Could you check a few things on this model? Use its own coordinates, in mm. Face numbers are marked on the shaded views. A direction names the side the tool comes from. Coordinates: 2 decimals unless noted, no trailing zeros. Loops run counter-clockwise (first coordinate to the right, second up) from the corner with the lowest first, then second, coordinate; pieces in that order, holes last. Notation, with made-up numbers: (16.5, 88.25) -> (40.5, 88.25) arc R15 ccw to (40.5, 98.25) -> close; hole circle Ø4 at (26, 0.5). An arc over 180 degrees is marked (long way). One line per question, with ' | ' between items. Start each with the question number.
(1) If we mould it in two halves opening along Z, with no side actions, what happens to the marked faces 1, 2 and 3? For each: pulls with the +Z half, pulls with the -Z half, needs draft (parallel to the pull), parting line crosses it, or undercut.
(2) Which directions (+Z, -Z, +X, -X, +Y, -Y) give clear straight access to the entire face, cutting with the end or side of a thin tool? Please do the marked faces 4 and 5.
(3) Suppose I cut it at B-B (y = 0). Please give me the cut outline in (x, z), plus the area to 3 significant figures.
(4) If I drill on line 1 along Z through (x, y) = (35.5, -33); line 2 along Z through (x, y) = (24.5, 41.5); line 3 along Y through (x, z) = (26.5, -79), over which ranges is the centre line in solid material (lowest first)?
(5) Suppose I cut it at A-A (x = 30). Give the number of separate pieces and of enclosed holes in the cut face, plus the area to 3 significant figures.
(6) I'm going to push flat-ended pins straight in: pin 1 Ø4 at (x, z) = (39.5, 85) entering from +Y; pin 2 Ø3 at (y, z) = (-20, 96) entering from -X; pin 3 Ø6 at (x, y) = (30.5, 65.5) entering from +Z; pin 4 Ø11 at (x, z) = (6.5, 47.5) entering from +Y. Where does each tip first touch, or does it pass through?
```python
from build123d import *

# Parameters (mm, degrees)
CUT_EXTRUDE1_START = -10
CUT_EXTRUDE1_DEPTH = 214.774440026
CUT_EXTRUDE2_DEPTH = 224.774440026


with BuildPart() as part:
    # Çizim1 → Döndür1 (revolve)
    with BuildSketch(Plane.XY, mode=Mode.PRIVATE) as d_nd_r1_sk:
        with BuildLine():
            Line((0, 31), (5, 31))
            Line((5, 31), (5, 32.75))
            Line((5, 32.75), (7.3, 32.75))
            Line((7.3, 32.75), (7.3, 31))
            Line((7.3, 31), (25, 31))
            Line((25, 31), (25, 16))
            Line((25, 16), (35, 16))
            Line((35, 16), (35, 0))
            Line((35, 0), (45, 0))
            Line((45, 0), (45, 148.5))
            Line((45, 148.5), (45, 150))
            ThreePointArc((45, 150), (43.535533906, 153.535533906), (40, 155))
            Line((40, 155), (25, 155))
            Line((25, 155), (25, 135))
            Line((25, 135), (5, 135))
            Line((5, 135), (0, 133))
            Line((0, 133), (0, 31))
        make_face()
    revolve(d_nd_r1_sk.sketch.rotate(Axis((0, 0, 0), (1, 0, 0)), 90), axis=Axis((0, 0, 0), (1, 0, 0)))

    # Sketch2 → Cut-Extrude1 (cut, through all)
    with BuildSketch(Plane.ZY.offset(CUT_EXTRUDE1_START)):
        with BuildLine():
            Line((82.068542495, 87.068542495), (31.068542495, 87.068542495))
            ThreePointArc((31.068542495, 87.068542495), (27.533008589, 85.604076401), (26.068542495, 82.068542495))
            Line((26.068542495, 82.068542495), (26.068542495, 31.068542495))
            ThreePointArc((26.068542495, 31.068542495), (27.533008589, 27.533008589), (31.068542495, 26.068542495))
            Line((31.068542495, 26.068542495), (82.068542495, 26.068542495))
            ThreePointArc((82.068542495, 26.068542495), (85.604076401, 27.533008589), (87.068542495, 31.068542495))
            Line((87.068542495, 31.068542495), (87.068542495, 82.068542495))
            ThreePointArc((87.068542495, 82.068542495), (85.604076401, 85.604076401), (82.068542495, 87.068542495))
        make_face()
        with BuildLine():
            Line((-82.068542495, 87.068542495), (-31.068542495, 87.068542495))
            ThreePointArc((-31.068542495, 87.068542495), (-27.533008589, 85.604076401), (-26.068542495, 82.068542495))
            Line((-26.068542495, 82.068542495), (-26.068542495, 31.068542495))
            ThreePointArc((-26.068542495, 31.068542495), (-27.533008589, 27.533008589), (-31.068542495, 26.068542495))
            Line((-31.068542495, 26.068542495), (-82.068542495, 26.068542495))
            ThreePointArc((-82.068542495, 26.068542495), (-85.604076401, 27.533008589), (-87.068542495, 31.068542495))
            Line((-87.068542495, 31.068542495), (-87.068542495, 82.068542495))
            ThreePointArc((-87.068542495, 82.068542495), (-85.604076401, 85.604076401), (-82.068542495, 87.068542495))
        make_face()
        with BuildLine():
            Line((87.068542495, -82.068542495), (87.068542495, -31.068542495))
            ThreePointArc((87.068542495, -31.068542495), (85.604076401, -27.533008589), (82.068542495, -26.068542495))
            Line((82.068542495, -26.068542495), (31.068542495, -26.068542495))
            ThreePointArc((31.068542495, -26.068542495), (27.533008589, -27.533008589), (26.068542495, -31.068542495))
            Line((26.068542495, -31.068542495), (26.068542495, -82.068542495))
            ThreePointArc((26.068542495, -82.068542495), (27.533008589, -85.604076401), (31.068542495, -87.068542495))
            Line((31.068542495, -87.068542495), (82.068542495, -87.068542495))
            ThreePointArc((82.068542495, -87.068542495), (85.604076401, -85.604076401), (87.068542495, -82.068542495))
        make_face()
        with BuildLine():
            Line((-82.068542495, -87.068542495), (-31.068542495, -87.068542495))
            ThreePointArc((-31.068542495, -87.068542495), (-27.533008589, -85.604076401), (-26.068542495, -82.068542495))
            Line((-26.068542495, -82.068542495), (-26.068542495, -31.068542495))
            ThreePointArc((-26.068542495, -31.068542495), (-27.533008589, -27.533008589), (-31.068542495, -26.068542495))
            Line((-31.068542495, -26.068542495), (-82.068542495, -26.068542495))
            ThreePointArc((-82.068542495, -26.068542495), (-85.604076401, -27.533008589), (-87.068542495, -31.068542495))
            Line((-87.068542495, -31.068542495), (-87.068542495, -82.068542495))
            ThreePointArc((-87.068542495, -82.068542495), (-85.604076401, -85.604076401), (-82.068542495, -87.068542495))
        make_face()
    extrude(amount=-CUT_EXTRUDE1_DEPTH, mode=Mode.SUBTRACT)

    # Sketch4 → Cut-Extrude2 (cut, through all)
    with BuildSketch(Plane.ZY):
        with BuildLine():
            Line((36.068542495, -31.068542495), (77.068542495, -31.068542495))
            ThreePointArc((77.068542495, -31.068542495), (80.604076401, -32.533008589), (82.068542495, -36.068542495))
            Line((82.068542495, -36.068542495), (82.068542495, -77.068542495))
            ThreePointArc((82.068542495, -77.068542495), (80.604076401, -80.604076401), (77.068542495, -82.068542495))
            Line((77.068542495, -82.068542495), (36.068542495, -82.068542495))
            ThreePointArc((36.068542495, -82.068542495), (32.533008589, -80.604076401), (31.068542495, -77.068542495))
            Line((31.068542495, -77.068542495), (31.068542495, -36.068542495))
            ThreePointArc((31.068542495, -36.068542495), (32.533008589, -32.533008589), (36.068542495, -31.068542495))
        make_face()
        with BuildLine():
            Line((-36.068542495, -31.068542495), (-77.068542495, -31.068542495))
            ThreePointArc((-77.068542495, -31.068542495), (-80.604076401, -32.533008589), (-82.068542495, -36.068542495))
            Line((-82.068542495, -36.068542495), (-82.068542495, -77.068542495))
            ThreePointArc((-82.068542495, -77.068542495), (-80.604076401, -80.604076401), (-77.068542495, -82.068542495))
            Line((-77.068542495, -82.068542495), (-36.068542495, -82.068542495))
            ThreePointArc((-36.068542495, -82.068542495), (-32.533008589, -80.604076401), (-31.068542495, -77.068542495))
            Line((-31.068542495, -77.068542495), (-31.068542495, -36.068542495))
            ThreePointArc((-31.068542495, -36.068542495), (-32.533008589, -32.533008589), (-36.068542495, -31.068542495))
        make_face()
        with BuildLine():
            Line((-31.068542495, 36.068542495), (-31.068542495, 77.068542495))
            ThreePointArc((-31.068542495, 77.068542495), (-32.533008589, 80.604076401), (-36.068542495, 82.068542495))
            Line((-36.068542495, 82.068542495), (-77.068542495, 82.068542495))
            ThreePointArc((-77.068542495, 82.068542495), (-80.604076401, 80.604076401), (-82.068542495, 77.068542495))
            Line((-82.068542495, 77.068542495), (-82.068542495, 36.068542495))
            ThreePointArc((-82.068542495, 36.068542495), (-80.604076401, 32.533008589), (-77.068542495, 31.068542495))
            Line((-77.068542495, 31.068542495), (-36.068542495, 31.068542495))
            ThreePointArc((-36.068542495, 31.068542495), (-32.533008589, 32.533008589), (-31.068542495, 36.068542495))
        make_face()
        with BuildLine():
            Line((36.068542495, 31.068542495), (77.068542495, 31.068542495))
            ThreePointArc((77.068542495, 31.068542495), (80.604076401, 32.533008589), (82.068542495, 36.068542495))
            Line((82.068542495, 36.068542495), (82.068542495, 77.068542495))
            ThreePointArc((82.068542495, 77.068542495), (80.604076401, 80.604076401), (77.068542495, 82.068542495))
            Line((77.068542495, 82.068542495), (36.068542495, 82.068542495))
            ThreePointArc((36.068542495, 82.068542495), (32.533008589, 80.604076401), (31.068542495, 77.068542495))
            Line((31.068542495, 77.068542495), (31.068542495, 36.068542495))
            ThreePointArc((31.068542495, 36.068542495), (32.533008589, 32.533008589), (36.068542495, 31.068542495))
        make_face()
    extrude(amount=-CUT_EXTRUDE2_DEPTH, mode=Mode.SUBTRACT)


solid = part.part
```
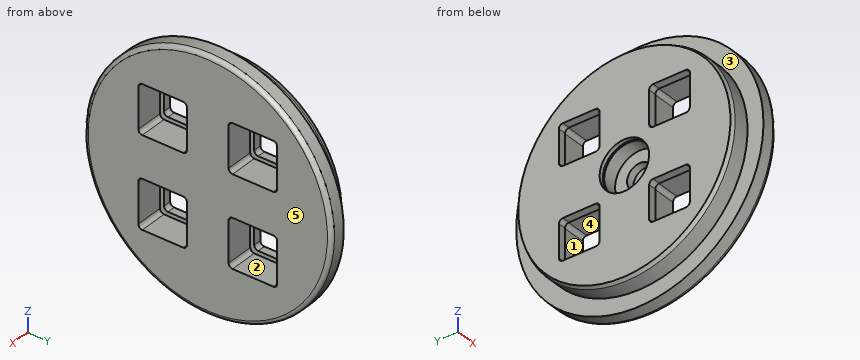
Checks:
1) face 1: undercut | face 2: undercut | face 3: needs draft
2) face 4: +X | face 5: +Z, -Z, +X, +Y, -Y
3) outline: (0, -133) -> (5, -135) -> (25, -135) -> (25, -155) -> (40, -155) arc R5 ccw to (45, -150) -> (45, 150) arc R5 ccw to (40, 155) -> (25, 155) -> (25, 135) -> (5, 135) -> (0, 133) -> (0, 31) -> (5, 31) -> (5, 32.75) -> (7.3, 32.75) -> (7.3, 31) -> (25, 31) -> (25, 16) -> (35, 16) -> (35, -16) -> (25, -16) -> (25, -31) -> (7.3, -31) -> (7.3, -32.75) -> (5, -32.75) -> (5, -31) -> (0, -31) -> close | area: 11,100 mm^2
4) line 1: z = -151.45 to -87.07, -26.07 to 26.07, 87.07 to 151.45 | line 2: z = -128.46 to -87.07, -26.07 to 26.07, 87.07 to 128.46 | line 3: y = -133.36 to -87.07, -26.07 to 26.07, 87.07 to 133.36
5) separate pieces: 1 | enclosed holes: 5 | area: 59,900 mm^2
6) pin 1: stops at y = 130.9 | pin 2: stops at x = 0 | pin 3: stops at z = 141.84 | pin 4: stops at y = 128.3
